Work out the finished part from the listing and answer in its coordinate system (mm). A direction names the side the tool comes from. Coordinates: 2 decimals unless noted, no trailing zeros. Loops run counter-clockwise (first coordinate to the right, second up) from the corner with the lowest first, then second, coordinate; pieces in that order, holes last.
```python
from build123d import *

# Parameters (mm, degrees)
F0_W     = 133.965507
F0_H     = 103.144266
F1_DEPTH = 25
F2_W     = 56.256611
F2_H     = 41.894164
F3_DEPTH = 10


with BuildPart() as f1:
    # F0 (on Front) → F1 (new body)
    with BuildSketch(Plane.XZ):
        with Locations((66.982754, 51.572133)):
            Rectangle(F0_W, F0_H)
    extrude(amount=-F1_DEPTH)

    # F2 (on Front) → F3 (join)
    with BuildSketch(Plane.XZ):
        with Locations((-28.128305, 20.947082)):
            Rectangle(F2_W, F2_H)
    extrude(amount=-F3_DEPTH)


solid = f1.part
```
1. A cutting plane is placed at D-D, the plane y = 2.25. Give the vertices of the cut face in (x, z), then the cut area to 3 significant figures.
2. A cutting plane is placed at A-A, the plane z = 31.5. Give the vertices of the cut face in (x, y).
3. Each of these flat-tipped pins is pushed along its axis until it touches: P1, Ø1, axis at y = 11, z = 68, coming from the -X side; P2, Ø5, axis at x = -19.5, y = 3.5, coming from the +Z side; P3, Ø12.5, axis at x = -27.5, z = 25, coming from the +Y side. Where does it stop, or does it pass through?
4. Straight lines are drawn through the part: probe 1 along X at (y, z) = (21.5, 75); probe 2 along Z at (x, y) = (-27, 3.5). For each, find the intervals that lie inside material, in ascending order.
5. For faces 1 (the flat face through (59, 0, 52)), 2 (the flat face through (-29, 10, 21)), 3 (the flat face through (-29, 5, 41.894)), determine the directions among +Z, -Z, +X, -X, +Y, -Y from which every point of the face is accessible in a straight line to the end or side of a thin tool.
6. A cutting plane is placed at C-C, the plane x = -5. Give the vertices of the cut face in (y, z), then the cut area to 3 significant figures.
7. A cutting plane is placed at B-B, the plane y = 16. Give the vertices of the cut face in (x, z), then the cut area to 3 significant figures.
Answers below:
1. outline: (-56.26, 0) - (133.97, 0) - (133.97, 103.14) - (0, 103.14) - (0, 41.89) - (-56.26, 41.89) - close
1. area: 16,200 mm2
2. outline: (-56.26, 0) - (133.97, 0) - (133.97, 25) - (0, 25) - (0, 10) - (-56.26, 10) - close
3. P1: stops at x = 0
3. P2: stops at z = 41.89
3. P3: stops at y = 10
4. probe 1: x = 0 to 133.97
4. probe 2: z = 0 to 41.89
5. face 1: +Z, -Z, +X, -X, -Y
5. face 2: +Z, -Z, -X, +Y
5. face 3: +Z, -X, +Y, -Y
6. outline: (0, 0) - (10, 0) - (10, 41.89) - (0, 41.89) - close
6. area: 419 mm2
7. outline: (0, 0) - (133.97, 0) - (133.97, 103.14) - (0, 103.14) - close
7. area: 13,800 mm2
